Source: CAD feature listing. Evaluate the final solid. Frame: model axes, mm. A direction names the side the tool comes from. Give positions to 0.01 mm unless a question says otherwise; leave off trailing zeros. Write each loop counter-clockwise with the first axis right and the second up, starting at its lowest first coordinate (ties: lowest second). Pieces come first, ordered by that corner, then holes. Notation, with made-up numbers: (16.25, 3) -> (33.25, 3) arc R34 cw to (33.25, 38) -> close; hole circle Ø1 at (57, 64.5). An arc over 180 degrees is marked (long way). Answer as a JSON object with one key per item and string values. Group by question number.
Item 1: Section query A-A on z = -80. Return the cut outline in (x, y), plus the area to 4 significant figures.
Item 2: First-contact query: pin 1 Ø1 at (x, y) = (571.5, 98) entering from -Z; pin 2 Ø10 at (x, y) = (442.5, 77) entering from +Z; pin 3 Ø12 at (x, y) = (474, 35.5) entering from +Z. Flat tips, straight axial feed; report the tip coordinate or a pass-through.
Item 3: Section query D-D on z = -17.5. Give the number of separate pieces and of enclosed holes in the cut face, plus the area to 3 significant figures.
Item 4: Pull-direction query (Y, two-part tool) for faces 1 (the face through (640, 99, -17)), 2 (the face through (79, 180, -81)), 3 (the face through (396, 45, -17)); classes: pulls with the +Y half, pulls with the -Y half, needs draft (parallel to the pull), parting line crosses it, or undercut.
Item 5: Access query for faces 4 (the face through (403, 20, -79)), 5 (the face through (437, 170, -137)), 6 (the face through (396, 155, -142)), 7 (the face through (632, 99, -25)), 8 (the face through (625, 38, -79)). Directions: +Z, -Z, +X, -X, +Y, -Y. A direction counts if a zero-diameter tool reaches every point of the face in a straight line with its end or side. Return the directions, or none.
Item 6: Section query B-B on y = 100. Return the cut outline in (x, z), plus the area to 4 significant figures.
Item 7: Section query C-C on x = 410. Return the cut outline in (y, z), plus the area to 3 significant figures.
Item 8: Ray query, probe 1 along Y at (x, z) = (595, -15.5); probe 2 along X at (y, z) = (31, -123); probe 3 along Y at (x, z) = (226.5, -104.5). Return the intervals inside material, ascending. Write a range as from..to.
from build123d import *

# Parameters (mm, degrees)
SKETCH1_W           = 640
SKETCH1_H           = 160
BOSS_EXTRUDE1_DEPTH = 180
SKETCH2_W           = 160
SKETCH2_H           = 160
CUT_EXTRUDE1_DEPTH  = 480
SKETCH3_R           = 70
BOSS_EXTRUDE2_DEPTH = 480
SKETCH4_W           = 15
SKETCH4_H           = 15
BOSS_EXTRUDE3_DEPTH = 480
SKETCH7_W           = 15
SKETCH7_H           = 15
BOSS_EXTRUDE4_DEPTH = 110
SKETCH8_W           = 15
SKETCH8_H           = 15
BOSS_EXTRUDE5_DEPTH = 110


with BuildPart() as part:
    # Sketch1 → Boss-Extrude1 (new body)
    with BuildSketch(Plane(origin=(0, 0, 0), x_dir=(1, 0, 0), z_dir=(0, 1, 0))):
        with Locations((320, 80)):
            Rectangle(SKETCH1_W, SKETCH1_H)
    extrude(amount=BOSS_EXTRUDE1_DEPTH)

    # Sketch2 → Cut-Extrude1 (cut)
    with BuildSketch(Plane(origin=(640, 0, 0), x_dir=(0, 0, -1), z_dir=(1, 0, 0))):
        with Locations((80, 100)):
            Rectangle(SKETCH2_W, SKETCH2_H)
    extrude(amount=-CUT_EXTRUDE1_DEPTH, mode=Mode.SUBTRACT)

    # Sketch3 → Boss-Extrude2 (add)
    with BuildSketch(Plane(origin=(160, 0, 0), x_dir=(0, 0, -1), z_dir=(1, 0, 0))):
        with Locations(Location((80, 100, 0), (0, 0, 180))):
            Circle(SKETCH3_R)
    extrude(amount=BOSS_EXTRUDE2_DEPTH)

    # Sketch6 → Cut-Revolve1 (revolve, cut)
    with BuildSketch(Plane.XY.offset(-80), mode=Mode.PRIVATE) as cut_revolve1_sk:
        Polygon((160, 170), (160, 150), (400, 170), align=None)
        Polygon((640, 150), (400, 170), (640, 170), align=None)
    revolve(cut_revolve1_sk.sketch.rotate(Axis((640, 100, -80), (-1, 0, 0)), 90), axis=Axis((640, 100, -80), (-1, 0, 0)), mode=Mode.SUBTRACT)

    # Sketch4 → Boss-Extrude3 (add)
    with BuildSketch(Plane(origin=(160, 0, 0), x_dir=(0, 0, -1), z_dir=(1, 0, 0))):
        with Locations((17.5, 162.5)):
            Rectangle(SKETCH4_W, SKETCH4_H)
        with Locations((142.5, 162.5)):
            Rectangle(SKETCH4_W, SKETCH4_H)
        with Locations((142.5, 37.5)):
            Rectangle(SKETCH4_W, SKETCH4_H)
        with Locations((17.5, 37.5)):
            Rectangle(SKETCH4_W, SKETCH4_H)
    extrude(amount=BOSS_EXTRUDE3_DEPTH)

    # Sketch7 → Boss-Extrude4 (add)
    with BuildSketch(Plane(origin=(0, 0, -25), x_dir=(-1, 0, 0), z_dir=(0, 0, -1))):
        with Locations((-632.5, 162.5)):
            Rectangle(SKETCH7_W, SKETCH7_H)
    boss_extrude4 = extrude(amount=BOSS_EXTRUDE4_DEPTH)

    # Mirror1: Boss-Extrude4 across plane
    add(boss_extrude4.mirror(Plane.ZX.offset(100)))

    # Sketch8 → Boss-Extrude5 (add)
    with BuildSketch(Plane(origin=(0, 45, 0), x_dir=(1, 0, 0), z_dir=(0, 1, 0))):
        with Locations((632.5, 17.5)):
            Rectangle(SKETCH8_W, SKETCH8_H)
        with Locations((632.5, 142.5)):
            Rectangle(SKETCH8_W, SKETCH8_H)
    extrude(amount=BOSS_EXTRUDE5_DEPTH)


solid = part.part
Worked answers:
{
 "1": {"outline": "(0, 0) -> (640, 0) -> (640, 20) -> (160, 20) -> (160, 50) -> (400, 30) -> (640, 50) -> (640, 150) -> (400, 170) -> (160, 150) -> (160, 180) -> (0, 180) -> close; (625, 30) -> (640, 30) -> (640, 45) -> (625, 45) -> close; (625, 155) -> (640, 155) -> (640, 170) -> (625, 170) -> close", "area": "96,450 mm^2"},
 "2": {"pin 1": "z = -135.72", "pin 2": "z = -15.96", "pin 3": "z = -10"},
 "3": {"separate pieces": "2", "enclosed holes": "1", "area": "61,900 mm^2"},
 "4": {"face 1": "needs draft", "face 2": "pulls with the +Y half", "face 3": "undercut"},
 "5": {"face 4": "+Z, -Z, +X", "face 5": "+Z, -Z, +X, +Y", "face 6": "-Z", "face 7": "+X", "face 8": "none"},
 "6": {"outline": "(0, -160) -> (160, -160) -> (160, -130) -> (400, -150) -> (640, -130) -> (640, -30) -> (400, -10) -> (160, -30) -> (160, 0) -> (0, 0) -> close; (625, -150) -> (640, -150) -> (640, -135) -> (625, -135) -> close; (625, -25) -> (640, -25) -> (640, -10) -> (625, -10) -> close", "area": "83,650 mm^2"},
 "7": {"outline": "(0, -160) -> (20, -160) -> (20, 0) -> (0, 0) -> close; (30, -150) -> (45, -150) -> (45, -135) -> (30, -135) -> close; (30, -25) -> (45, -25) -> (45, -10) -> (30, -10) -> close; circle Ø138.33 at (100, -80); (155, -150) -> (170, -150) -> (170, -135) -> (155, -135) -> close; (155, -25) -> (170, -25) -> (170, -10) -> (155, -10) -> close", "area": "19,100 mm^2"},
 "8": {"probe 1": "0..20, 30..45, 155..170", "probe 2": "0..160, 625..640", "probe 3": "0..20, 50.15..149.85"}
}
